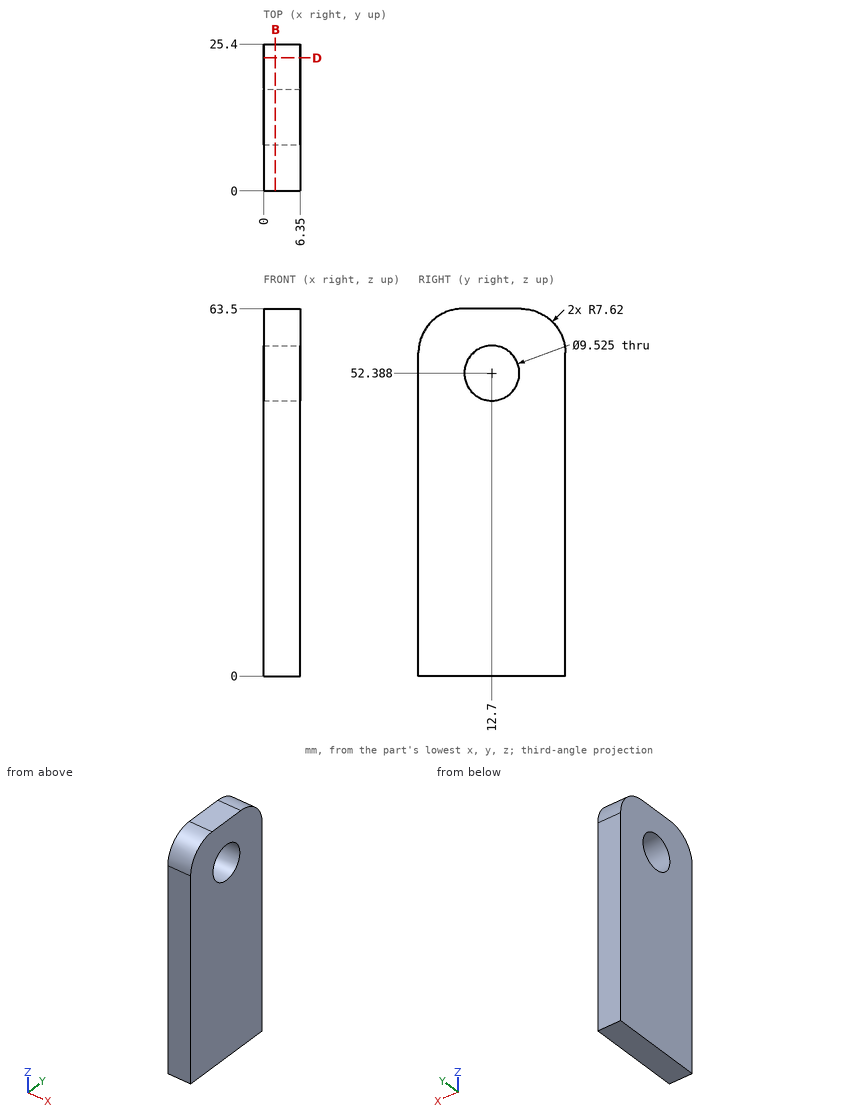
Geometry check sheet. Reference: drawing and pictorial views, mm from the part's lowest x, y, z. Round coordinates to 2 decimals unless told otherwise and drop trailing zeros. Loops run counter-clockwise (first coordinate to the right, second up) from the corner with the lowest first, then second, coordinate; pieces in that order, holes last. Notation, with made-up numbers: M 89,3 L 109,3 A21 ccw 109,22 Z; hole C 22.5,70 d6. An arc over 180 degrees is marked long. One line per item, written item: value.
(1) Sectioned sample at D-D, the plane y = 23. Record the cut outline in (x, z).
Computed values:
outline: M 0,0 L 6.35,0 L 6.35,61.43 L 0,61.43 Z
(2) Thickness scan on line 1 (Z direction, x = 5.25, y = 12.5) (1 decimal); line 2 (Y direction, x = 5.5, z = 50); line 3 (Z direction, x = 3, y = 14.5) (1 decimal). Record the ranges inside material, lowest first.
Computed values:
line 1: z = 0 to 47.6, 57.1 to 63.5
line 2: y = 0 to 8.58, 16.82 to 25.4
line 3: z = 0 to 48, 56.8 to 63.5
(3) Depth check by flat-ended pin: pin 1 Ø1.5 at (y, z) = (13, 49) entering from -X. Enter the tip coordinate at first touch or a pass-through.
Computed values:
pin 1: passes through
(4) Sectioned sample at B-B, the plane x = 2. Record the cut outline in (y, z) (1 decimal), then the cut area to 3 significant figures.
Computed values:
outline: M 0,0 L 25.4,0 L 25.4,55.9 A7.6 ccw 17.8,63.5 L 7.6,63.5 A7.6 ccw 0,55.9 Z; hole C 12.7,52.4 d9.5
area: 1,520 mm^2
